from build123d import *

# Parameters (mm, degrees)
SKETCH1_R               = 88.9
SKETCH1_R_2             = 82.55
BOSS_EXTRUDE1_DEPTH     = 25.4
SKETCH2_R               = 2.413
CUT_EXTRUDE1_DEPTH      = 89.9
CUT_EXTRUDE1_DEPTH_BACK = 89.9
SKETCH3_R               = 2.159
CUT_EXTRUDE2_DEPTH      = 89.9000001
CUT_EXTRUDE2_DEPTH_BACK = 89.9000001


with BuildPart() as part:
    # Sketch1 → Boss-Extrude1 (new body)
    with BuildSketch(Plane(origin=(0, 0, 0), x_dir=(1, 0, 0), z_dir=(0, 1, 0))):
        Circle(SKETCH1_R)
        Circle(SKETCH1_R_2, mode=Mode.SUBTRACT)
    extrude(amount=BOSS_EXTRUDE1_DEPTH)

    # Sketch2 → Cut-Extrude1 (cut, two sides)
    with BuildSketch(Plane(origin=(0, 0, 0), x_dir=(0, 0, -1), z_dir=(1, 0, 0))) as cut_extrude1_sk:
        with Locations((0, 12.7)):
            Circle(SKETCH2_R)
    extrude(amount=CUT_EXTRUDE1_DEPTH, mode=Mode.SUBTRACT)
    extrude(cut_extrude1_sk.sketch, amount=-CUT_EXTRUDE1_DEPTH_BACK, mode=Mode.SUBTRACT)

    # Sketch3 → Cut-Extrude2 (cut, two sides)
    with BuildSketch(Plane.XY) as cut_extrude2_sk:
        with Locations((0, 12.7)):
            Circle(SKETCH3_R)
    extrude(amount=CUT_EXTRUDE2_DEPTH, mode=Mode.SUBTRACT)
    extrude(cut_extrude2_sk.sketch, amount=-CUT_EXTRUDE2_DEPTH_BACK, mode=Mode.SUBTRACT)


solid = part.part
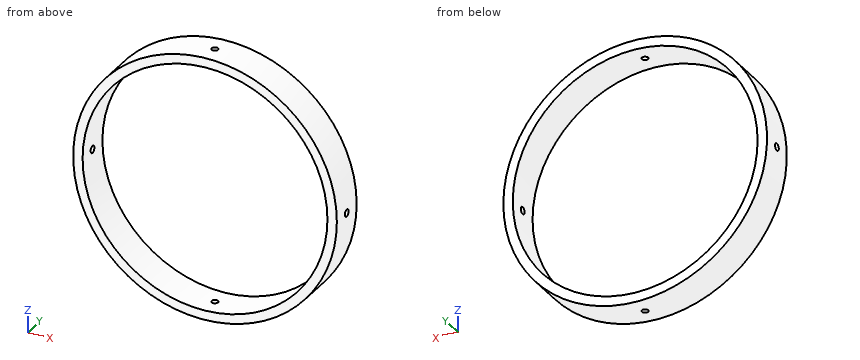
The model under review builds one solid part; all positions refer to its coordinate system, in mm. Give positions to 0.01 mm unless a question says otherwise; leave off trailing zeros. Write each loop counter-clockwise with the first axis right and the second up, starting at its lowest first coordinate (ties: lowest second). Pieces come first, ordered by that corner, then holes.
1. Add section B-B, the plane y = 12.7. Write out the cut boundary in (x, z).
2. Add section D-D, the plane z = 34.5. Write out the cut boundary in (x, y), plus the area to 3 significant figures.
3. Add section C-C, the plane x = 41. Write out the cut boundary in (y, z), plus the area to 3 significant figures.
4. Add section A-A, the plane z = 0. Write out the cut boundary in (x, y), plus the area to 3 significant figures.
5. Wall thickness on L1, parallel to Y at x = 87, z = 0; L2, parallel to Y at x = 0, z = -86.75; L3, parallel to X at y = 21.25, z = -1: over which ranges is each line inside the solid? List them lowest first.
6. For P1, Ø5, axis at x = -17, y = 8, coming from the +Z side; P2, Ø8, axis at y = 15, z = -57, coming from the -X side; P3, Ø8, axis at y = 14.5, z = -48, coming from the -X side, all flat-tipped, find the tip position at first contact; note any pin that passes through.
Worked answers:
1. outline: (-88.87, -2.41) arc R88.9 ccw to (-2.16, -88.87) - (-2.16, -82.52) arc R82.55 cw to (-82.51, -2.41) - close; (-88.87, 2.41) - (-82.51, 2.41) arc R82.55 cw to (-2.16, 82.52) - (-2.16, 88.87) arc R88.9 ccw to start; (2.16, -88.87) arc R88.9 ccw to (88.87, -2.41) - (82.51, -2.41) arc R82.55 cw to (2.16, -82.52) - close; (2.16, 82.52) arc R82.55 cw to (82.51, 2.41) - (88.87, 2.41) arc R88.9 ccw to (2.16, 88.87) - close
2. outline: (-81.93, 0) - (-75, 0) - (-75, 25.4) - (-81.93, 25.4) - close; (75, 0) - (81.93, 0) - (81.93, 25.4) - (75, 25.4) - close
2. area: 352 mm2
3. outline: (0, -78.88) - (25.4, -78.88) - (25.4, -71.65) - (0, -71.65) - close; (0, 71.65) - (25.4, 71.65) - (25.4, 78.88) - (0, 78.88) - close
3. area: 367 mm2
4. outline: (-88.9, 0) - (-82.55, 0) - (-82.55, 10.29) - (-88.9, 10.29) - close; (-88.9, 15.11) - (-82.55, 15.11) - (-82.55, 25.4) - (-88.9, 25.4) - close; (82.55, 0) - (88.9, 0) - (88.9, 10.29) - (82.55, 10.29) - close; (82.55, 15.11) - (88.9, 15.11) - (88.9, 25.4) - (82.55, 25.4) - close
4. area: 261 mm2
5. L1: y = 0 to 10.29, 15.11 to 25.4
5. L2: y = 0 to 10.54, 14.86 to 25.4
5. L3: x = -88.89 to -82.54, 82.54 to 88.89
6. P1: stops at z = 87.71
6. P2: stops at x = -71.37
6. P3: stops at x = -77.25
